CAD build for the part. Positions are in the model's coordinates, mm. A direction names the side the tool comes from. Give positions to 0.01 mm unless a question says otherwise; leave off trailing zeros. Use one line per item in the form item = value. Start each with the question number.
1) Probe line 1 (X direction, y = 43.5, z = -2.25); line 2 (Y direction, x = 24, z = 2.75); line 3 (Y direction, x = 45, z = -3.75). List the from-to ranges inside material, lowest first.
2) Mould opens along X. For faces 3 (the face through (16.021, 50.025, 0.07)), 4 (the face through (31.973, 34.287, 0.07)) say: pulls with the +X half, pulls with the -X half, needs draft (parallel to the pull), parting line crosses it, or undercut.
3) Tool access for faces 1 (the face through (5, 45, 4)), 2 (the face through (38.64, 35.58, 0.07)): list every direction of +Z, -Z, +X, -X, +Y, -Y with a clear straight run to the whole face (end or side of a thin tool).
4) Drop flat-ended pins along their axis: P1, Ø1.5, axis at x = 21, z = -2.5, coming from the +Y side; P2, Ø4, axis at x = 35.5, z = -3.5, coming from the +Y side; P3, Ø5, axis at x = 14.5, z = 1.5, coming from the -Y side. Give the stop position or say it passes through.
from build123d import *

# Parameters (mm, degrees)
AUFSATZ_LINEAR_AUSTRAGEN1_DEPTH = 5
AUFSATZ_LINEAR_AUSTRAGEN2_DEPTH = 5
KREISMUSTER1_COUNT              = 11
KREISMUSTER1_ANGLE              = 74
AUFSATZ_LINEAR_AUSTRAGEN3_DEPTH = 5
AUFSATZ_LINEAR_AUSTRAGEN4_DEPTH = 1
KREISMUSTER2_COUNT              = 10
KREISMUSTER2_ANGLE              = 66.6
KREISMUSTER2_COPY_1_DEPTH       = 1
KREISMUSTER2_COPY_2_DEPTH       = 1
KREISMUSTER2_COPY_3_DEPTH       = 1
KREISMUSTER2_COPY_4_DEPTH       = 1
KREISMUSTER2_COPY_5_DEPTH       = 1
KREISMUSTER2_COPY_6_DEPTH       = 1
KREISMUSTER2_COPY_7_DEPTH       = 1
KREISMUSTER2_COPY_8_DEPTH       = 1
KREISMUSTER2_COPY_9_DEPTH       = 1


with BuildPart() as part:
    # Skizze1 → Aufsatz-Linear austragen1 (new, symmetric)
    with BuildSketch(Plane.XY):
        with BuildLine():
            Line((0, 41), (0, 40))
            ThreePointArc((0, 40), (25.711504387, 30.641777725), (39.39231012, 6.945927107))
            Line((39.39231012, 6.945927107), (40.377117874, 7.119575284))
            ThreePointArc((40.377117874, 7.119575284), (26.354291997, 31.407822168), (0, 41))
        make_face()
    extrude(amount=AUFSATZ_LINEAR_AUSTRAGEN1_DEPTH, both=True)

    # Skizze2 → Aufsatz-Linear austragen2 (add, symmetric)
    with BuildSketch(Plane.XY):
        with BuildLine():
            Line((0, 41), (0, 52.6))
            Line((0, 52.6), (5.498197168, 52.311851696))
            Line((5.498197168, 52.311851696), (4.285666994, 40.77539771))
            ThreePointArc((4.285666994, 40.77539771), (2.145774206, 40.943810925), (0, 41))
        make_face()
    aufsatz_linear_austragen2 = extrude(amount=AUFSATZ_LINEAR_AUSTRAGEN2_DEPTH, both=True)

    # Kreismuster1: Aufsatz-Linear austragen2 ×11 about axis
    kreismuster1_axis = Axis((0, 0, 0), (0, 0, -1))
    for i in range(1, KREISMUSTER1_COUNT):
        add(aufsatz_linear_austragen2.rotate(kreismuster1_axis, i * KREISMUSTER1_ANGLE / (KREISMUSTER1_COUNT - 1)))

    # Skizze3 → Aufsatz-Linear austragen3 (add, symmetric)
    with BuildSketch(Plane.XY):
        with BuildLine():
            ThreePointArc((38.407502367, 6.772278929), (25.068716778, 29.875733282), (0, 39))
            Line((0, 39), (0, 40))
            ThreePointArc((0, 40), (25.711504387, 30.641777725), (39.39231012, 6.945927107))
            Line((39.39231012, 6.945927107), (38.407502367, 6.772278929))
        make_face()
    extrude(amount=AUFSATZ_LINEAR_AUSTRAGEN3_DEPTH, both=True)

    # Skizze4 → Aufsatz-Linear austragen4 (add)
    with BuildSketch(Plane(origin=(0, 0, -5), x_dir=(-1, 0, 0), z_dir=(0, 0, -1))):
        with BuildLine():
            Line((-47.678364885, 13.671551131), (-39.411729533, 11.301131588))
            Line((-39.411729533, 11.301131588), (-39.123853469, 12.260672482))
            Line((-39.123853469, 12.260672482), (-47.330106633, 14.832356338))
            ThreePointArc((-47.330106633, 14.832356338), (-47.149949209, 14.145662676), (-47.678364885, 13.671551131))
        make_face()
    aufsatz_linear_austragen4 = extrude(amount=-AUFSATZ_LINEAR_AUSTRAGEN4_DEPTH)

    # Spiegeln1: Aufsatz-Linear austragen4 across plane
    add(aufsatz_linear_austragen4.mirror(Plane.XY))

    # Kreismuster2: Aufsatz-Linear austragen4 ×10 about axis
    kreismuster2_axis = Axis((0, 0, 0), (0, 0, 1))
    for i in range(1, KREISMUSTER2_COUNT):
        add(aufsatz_linear_austragen4.rotate(kreismuster2_axis, i * KREISMUSTER2_ANGLE / (KREISMUSTER2_COUNT - 1)))

    # Kreismuster2 copy 1 sketch → Kreismuster2 copy 1 (add)
    with BuildSketch(Plane(origin=(0, 0, 5), x_dir=(-0.9916711623830904, -0.12879559657756307, 0), z_dir=(0, 0, 1))):
        with BuildLine():
            Line((-47.678364885, -13.671551131), (-39.411729533, -11.301131588))
            Line((-39.411729533, -11.301131588), (-39.123853469, -12.260672482))
            Line((-39.123853469, -12.260672482), (-47.330106633, -14.832356338))
            ThreePointArc((-47.330106633, -14.832356338), (-47.149949209, -14.145662676), (-47.678364885, -13.671551131))
        make_face()
    extrude(amount=-KREISMUSTER2_COPY_1_DEPTH)

    # Kreismuster2 copy 2 sketch → Kreismuster2 copy 2 (add)
    with BuildSketch(Plane(origin=(0, 0, 5), x_dir=(-0.9668233886044593, -0.2554457579357911, 0), z_dir=(0, 0, 1))):
        with BuildLine():
            Line((-47.678364885, -13.671551131), (-39.411729533, -11.301131588))
            Line((-39.411729533, -11.301131588), (-39.123853469, -12.260672482))
            Line((-39.123853469, -12.260672482), (-47.330106633, -14.832356338))
            ThreePointArc((-47.330106633, -14.832356338), (-47.149949209, -14.145662676), (-47.678364885, -13.671551131))
        make_face()
    extrude(amount=-KREISMUSTER2_COPY_2_DEPTH)

    # Kreismuster2 copy 3 sketch → Kreismuster2 copy 3 (add)
    with BuildSketch(Plane(origin=(0, 0, 5), x_dir=(-0.9258705848099944, -0.37784078681846794, 0), z_dir=(0, 0, 1))):
        with BuildLine():
            Line((-47.678364885, -13.671551131), (-39.411729533, -11.301131588))
            Line((-39.411729533, -11.301131588), (-39.123853469, -12.260672482))
            Line((-39.123853469, -12.260672482), (-47.330106633, -14.832356338))
            ThreePointArc((-47.330106633, -14.832356338), (-47.149949209, -14.145662676), (-47.678364885, -13.671551131))
        make_face()
    extrude(amount=-KREISMUSTER2_COPY_3_DEPTH)

    # Kreismuster2 copy 4 sketch → Kreismuster2 copy 4 (add)
    with BuildSketch(Plane(origin=(0, 0, 5), x_dir=(-0.8694949295052185, -0.493941866584232, 0), z_dir=(0, 0, 1))):
        with BuildLine():
            Line((-47.678364885, -13.671551131), (-39.411729533, -11.301131588))
            Line((-39.411729533, -11.301131588), (-39.123853469, -12.260672482))
            Line((-39.123853469, -12.260672482), (-47.330106633, -14.832356338))
            ThreePointArc((-47.330106633, -14.832356338), (-47.149949209, -14.145662676), (-47.678364885, -13.671551131))
        make_face()
    extrude(amount=-KREISMUSTER2_COPY_4_DEPTH)

    # Kreismuster2 copy 5 sketch → Kreismuster2 copy 5 (add)
    with BuildSketch(Plane(origin=(0, 0, 5), x_dir=(-0.7986355100472919, -0.6018150231520494, 0), z_dir=(0, 0, 1))):
        with BuildLine():
            Line((-47.678364885, -13.671551131), (-39.411729533, -11.301131588))
            Line((-39.411729533, -11.301131588), (-39.123853469, -12.260672482))
            Line((-39.123853469, -12.260672482), (-47.330106633, -14.832356338))
            ThreePointArc((-47.330106633, -14.832356338), (-47.149949209, -14.145662676), (-47.678364885, -13.671551131))
        make_face()
    extrude(amount=-KREISMUSTER2_COPY_5_DEPTH)

    # Kreismuster2 copy 6 sketch → Kreismuster2 copy 6 (add)
    with BuildSketch(Plane(origin=(0, 0, 5), x_dir=(-0.7144726796328021, -0.6996633405133666, 0), z_dir=(0, 0, 1))):
        with BuildLine():
            Line((-47.678364885, -13.671551131), (-39.411729533, -11.301131588))
            Line((-39.411729533, -11.301131588), (-39.123853469, -12.260672482))
            Line((-39.123853469, -12.260672482), (-47.330106633, -14.832356338))
            ThreePointArc((-47.330106633, -14.832356338), (-47.149949209, -14.145662676), (-47.678364885, -13.671551131))
        make_face()
    extrude(amount=-KREISMUSTER2_COPY_6_DEPTH)

    # Kreismuster2 copy 7 sketch → Kreismuster2 copy 7 (add)
    with BuildSketch(Plane(origin=(0, 0, 5), x_dir=(-0.6184083953575527, -0.7858568931754031, 0), z_dir=(0, 0, 1))):
        with BuildLine():
            Line((-47.678364885, -13.671551131), (-39.411729533, -11.301131588))
            Line((-39.411729533, -11.301131588), (-39.123853469, -12.260672482))
            Line((-39.123853469, -12.260672482), (-47.330106633, -14.832356338))
            ThreePointArc((-47.330106633, -14.832356338), (-47.149949209, -14.145662676), (-47.678364885, -13.671551131))
        make_face()
    extrude(amount=-KREISMUSTER2_COPY_7_DEPTH)

    # Kreismuster2 copy 8 sketch → Kreismuster2 copy 8 (add)
    with BuildSketch(Plane(origin=(0, 0, 5), x_dir=(-0.5120428648705696, -0.8589598969306655, 0), z_dir=(0, 0, 1))):
        with BuildLine():
            Line((-47.678364885, -13.671551131), (-39.411729533, -11.301131588))
            Line((-39.411729533, -11.301131588), (-39.123853469, -12.260672482))
            Line((-39.123853469, -12.260672482), (-47.330106633, -14.832356338))
            ThreePointArc((-47.330106633, -14.832356338), (-47.149949209, -14.145662676), (-47.678364885, -13.671551131))
        make_face()
    extrude(amount=-KREISMUSTER2_COPY_8_DEPTH)

    # Kreismuster2 copy 9 sketch → Kreismuster2 copy 9 (add)
    with BuildSketch(Plane(origin=(0, 0, 5), x_dir=(-0.3971478906347781, -0.9177546256839823, 0), z_dir=(0, 0, 1))):
        with BuildLine():
            Line((-47.678364885, -13.671551131), (-39.411729533, -11.301131588))
            Line((-39.411729533, -11.301131588), (-39.123853469, -12.260672482))
            Line((-39.123853469, -12.260672482), (-47.330106633, -14.832356338))
            ThreePointArc((-47.330106633, -14.832356338), (-47.149949209, -14.145662676), (-47.678364885, -13.671551131))
        make_face()
    extrude(amount=-KREISMUSTER2_COPY_9_DEPTH)


solid = part.part
Result:
q1.line_1 = 0 to 4.57, 5.65 to 10.36, 11.49 to 16.52, 17.75 to 23.32, 24.71 to 29.48
q1.line_2 = 30.74 to 33.24, 33.52 to 42.25, 44.76 to 46.76
q1.line_3 = 7.93 to 12.9, 14.1 to 19.47, 20.79 to 26.83
q2.face_3 = pulls with the +X half
q2.face_4 = undercut
q3.face_1 = none
q3.face_2 = +Z, -Z, +X, +Y
q4.P1 = 48.52
q4.P2 = 40.46
q4.P3 = 35.1
